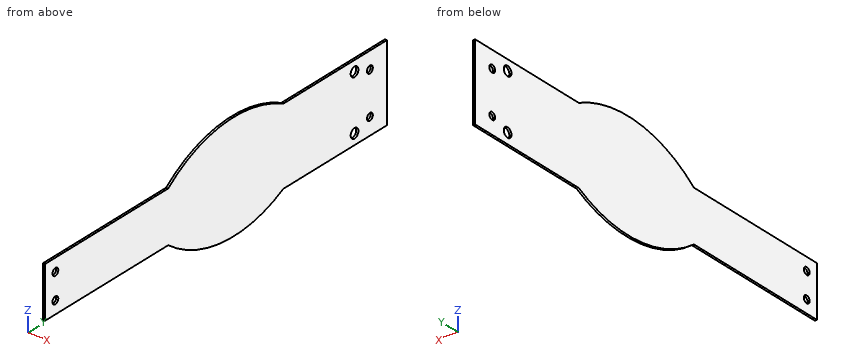
from build123d import *

# Parameters (mm, degrees)
BOSS_EXTRUDE1_DEPTH  = 1
M4_CLEARANCE_HOLE1_D = 4.5
M3_CLEARANCE_HOLE1_D = 3.4
M3_CLEARANCE_HOLE2_D = 3.4


with BuildPart() as part:
    # Sketch1 → Boss-Extrude1 (new body)
    with BuildSketch(Plane(origin=(0, 0, 0), x_dir=(0, 0, -1), z_dir=(1, 0, 0))):
        with BuildLine():
            Line((12, -200), (12, -128))
            ThreePointArc((12, -128), (25, -95.198992339), (18, -60.617116977))
            Line((18, -60.617116977), (18, 0))
            Line((18, 0), (-18, 0))
            Line((-18, 0), (-18, -60.617116977))
            ThreePointArc((-18, -60.617116977), (-25, -95.198992339), (-12, -128))
            Line((-12, -128), (-12, -200))
            Line((-12, -200), (12, -200))
        make_face()
    extrude(amount=BOSS_EXTRUDE1_DEPTH)

    # M4 Clearance Hole1 (through all)
    with Locations(Plane.ZY):
        with Locations((13, -19), (-13, -19)):
            Hole(M4_CLEARANCE_HOLE1_D / 2)

    # M3 Clearance Hole1 (through all)
    with Locations(Plane.ZY):
        with Locations((-10, -10), (10, -10)):
            Hole(M3_CLEARANCE_HOLE1_D / 2)

    # M3 Clearance Hole2 (through all)
    with Locations(Plane.ZY):
        with Locations((6, -194), (-6, -194)):
            Hole(M3_CLEARANCE_HOLE2_D / 2)


solid = part.part
The listing builds one solid part. Answer for the finished solid, in the listing's coordinates (mm). Round coordinates to 2 decimals unless told otherwise and drop trailing zeros. Write each loop counter-clockwise with the first axis right and the second up, starting at its lowest first coordinate (ties: lowest second). Pieces come first, ordered by that corner, then holes. Notation, with made-up numbers: (75, 26) - (98, 26) arc R28 cw to (98, 55) - close; hole circle Ø7 at (44.25, -26.75). An arc over 180 degrees is marked (long way). Use one line per item in the form item = value. Start each with the question number.
Item 1: A cutting plane is placed at A-A (y = -194). Write down the section's boundary in (x, z), plus the area to 3 significant figures.
Item 2: A cutting plane is placed at B-B (z = 6). Write down the section's boundary in (x, y).
Item 3: Flat-ended cylindrical pins translate along their axes: pin 1 Ø5 at (y, z) = (-19, -13) entering from +X; pin 2 Ø0.5 at (x, y) = (0.5, -31.5) entering from -Z; pin 3 Ø3 at (y, z) = (-194, 6) entering from -X. Find the tip coordinate at first contact, or state that the pin passes through.
Item 4: Find the intervals of material crossed by line 1 (Z direction, x = 0.65, y = -194); line 2 (Y direction, x = 0.3, z = 6); line 3 (Z direction, x = 0.3, y = -163), in increasing order. Write a range as [from, to].
Item 5: A cutting plane is placed at D-D (y = -133.5). Write down the section's boundary in (x, z), plus the area to 3 significant figures.
Item 6: A cutting plane is placed at C-C (x = 0.4). Write down the section's boundary in (y, z), plus the area to 3 significant figures.
The answers:
q1.outline = (0, -12) - (1, -12) - (1, -7.7) - (0, -7.7) - close; (0, -4.3) - (1, -4.3) - (1, 4.3) - (0, 4.3) - close; (0, 7.7) - (1, 7.7) - (1, 12) - (0, 12) - close
q1.area = 17.2 mm^2
q2.outline = (0, -200) - (1, -200) - (1, -195.7) - (0, -195.7) - close; (0, -192.3) - (1, -192.3) - (1, 0) - (0, 0) - close
q3.pin_1 = 1
q3.pin_2 = -18
q3.pin_3 = through
q4.line_1 = [-12, -7.7], [-4.3, 4.3], [7.7, 12]
q4.line_2 = [-200, -195.7], [-192.3, 0]
q4.line_3 = [-12, 12]
q5.outline = (0, -12) - (1, -12) - (1, 12) - (0, 12) - close
q5.area = 24.0 mm^2
q6.outline = (-200, -12) - (-128, -12) arc R62 ccw to (-60.62, -18) - (0, -18) - (0, 18) - (-60.62, 18) arc R62 ccw to (-128, 12) - (-200, 12) - close; hole circle Ø3.4 at (-194, -6); hole circle Ø3.4 at (-194, 6); hole circle Ø4.5 at (-19, -13); hole circle Ø4.5 at (-19, 13); hole circle Ø3.4 at (-10, -10); hole circle Ø3.4 at (-10, 10)
q6.area = 6,780 mm^2
